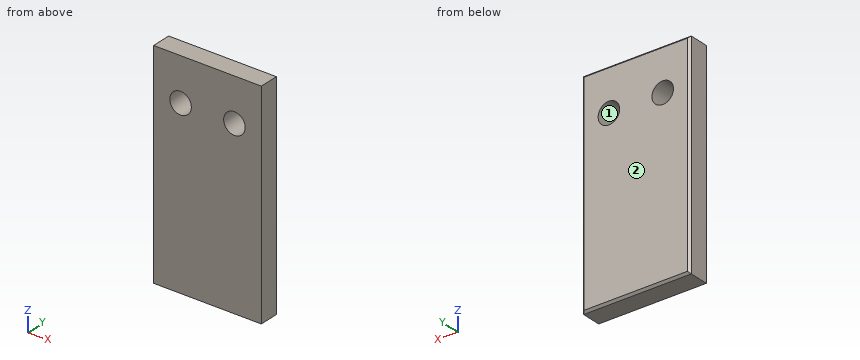
Autodesk Inventor part; units mm, degrees
ref_plane "YZ Plane" through (0, 0, 0) normal (1, 0, 0) x (0, 1, 0)
ref_plane "XZ Plane" through (0, 0, 0) normal (0, 1, 0) x (-1, 0, 0)
ref_plane "XY Plane" through (0, 0, 0) normal (0, 0, 1) x (1, 0, 0)
sketch "草圖1" plane through (0, 0, 0) normal (0, 1, 0) x (-1, 0, 0)
  line L0 (25, 50) -> (-25, 50)
  line L1 (-25, 50) -> (-25, -50)
  line L2 (-25, -50) -> (25, -50)
  line L3 (25, -50) -> (25, 50)
  circle A0 centre (12.5, 30) radius 5
  circle A1 centre (-12.5, 30) radius 5
  point P0 (0, 0)
  point P1 (25, 0)
  point P2 (0, -50)
  dimension "d0" = 50
  dimension "d1" = 100
  dimension "d2" = 25
  dimension "d3" = 12.5
  dimension "d4" = 10
  dimension "d5" = 20
extrude "擠出1" add sketch "草圖1" along normal blind 10
chamfer "倒角1" distance 1 angle 45 4 edges at (0, 10, 50) (-25, 10, 0) (25, 10, 0) (0, 10, -50)
thread "螺紋1"
thread "螺紋2"
properties part number "P10"
Geometry: final body of the model. Coordinates: model frame, mm. Face numbers are marked on the shaded views. Coordinates: 2 decimals unless noted, no trailing zeros. Write each loop counter-clockwise with the first axis right and the second up, starting at its lowest first coordinate (ties: lowest second). Pieces come first, ordered by that corner, then holes. Notation, with made-up numbers: (-28.5, -9.5) - (-12.5, -9.5) arc R14 ccw to (-12.5, 14.5) - close; hole circle Ø4 at (-3.5, 51). An arc over 180 degrees is marked (long way). Return JSON: item names as keys, results as strings.
Item 1: Section query C-C (y = 6.5). Output: boundary loops of the cut face in (x, z), and give its area (3 significant figures).
Completed:
{"outline": "(-25, -50) - (25, -50) - (25, 50) - (-25, 50) - close; hole circle Ø10 at (-12.5, 30); hole circle Ø10 at (12.5, 30)", "area": "4,840 mm2"}
Item 2: Section query B-B (z = 30). Output: boundary loops of the cut face in (x, y).
Completed:
{"outline": "(-25, 0) - (-17.5, 0) - (-17.5, 10) - (-24, 10) - (-25, 9) - close; (-7.5, 0) - (7.5, 0) - (7.5, 10) - (-7.5, 10) - close; (17.5, 0) - (25, 0) - (25, 9) - (24, 10) - (17.5, 10) - close"}
Item 3: Pull-direction query (X, two-part tool) for the marked faces 1 and 2; classes: +X half, -X half, draft (parallel to the pull), parting line (faces both ways), or undercut.
Completed:
{"face 1": "undercut", "face 2": "draft"}
Item 4: Section query A-A (x = -12.5). Output: boundary loops of the cut face in (y, z), and give its area (3 significant figures).
Completed:
{"outline": "(0, -50) - (9, -50) - (10, -49) - (10, 25) - (0, 25) - close; (0, 35) - (10, 35) - (10, 49) - (9, 50) - (0, 50) - close", "area": "899 mm2"}
Item 5: Line query: L1, parallel to Z at x = -12.5, y = 4.25; L2, parallel to Z at x = -14.5, y = 6; L3, parallel to X at y = 9.75, z = -15. Output: solid intervals per line, ascending.
Completed:
{"L1": "z = -50 to 25, 35 to 50", "L2": "z = -50 to 25.42, 34.58 to 50", "L3": "x = -24.25 to 24.25"}
